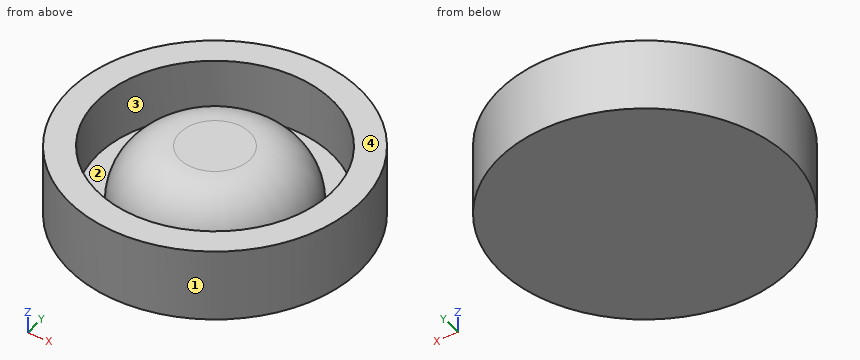
```python
from build123d import *

# Parameters (mm, degrees)
F0_R     = 25.4
F1_DEPTH = 12.7
F2_R     = 20.5279895556
F3_DEPTH = 10.16
F4_R     = 16.2758477469
F5_DEPTH = 10.16
F6_R     = 10.15999


# Not quite as in the source:
# - a fillet or chamfer is up to 0.001 mm smaller than in the source, because OpenCascade refuses the exact size


with BuildPart() as f1:
    # F0 (on Top) → F1 (new body)
    with BuildSketch(Plane.XY):
        Circle(F0_R)
    extrude(amount=F1_DEPTH)

    # F2 (on face) → F3 (cut)
    with BuildSketch(Plane.XY.offset(12.7)):
        Circle(F2_R)
    extrude(amount=-F3_DEPTH, mode=Mode.SUBTRACT)

    # F4 (on face) → F5 (join)
    with BuildSketch(Plane.XY.offset(2.54)):
        Circle(F4_R)
    extrude(amount=F5_DEPTH)

    # F6 (radius 10.16 in the source; OpenCascade refuses exactly that, so slightly less here)
    f6_edges = [f1.edges().sort_by_distance(p)[0] for p in [
        (-16.275848, 0, 12.7),
    ]]
    fillet(f6_edges, radius=F6_R)


solid = f1.part
```
For this review, take the finished solid that the model builds, in its own axes (mm). Face numbers are marked on the shaded views. Round coordinates to 2 decimals unless told otherwise and drop trailing zeros. Loops run counter-clockwise (first coordinate to the right, second up) from the corner with the lowest first, then second, coordinate; pieces in that order, holes last.
Q1. Mouldability with a two-part tool opening along Y and no side actions: class the marked faces 1, 2, 3 and 4 as +Y half, -Y half, draft (parallel to the pull), parting line (faces both ways), or undercut.
Result sheet:
face 1: parting line
face 2: undercut
face 3: undercut
face 4: draft
Q2. Insertion check: pin 1 Ø8 at (x, y) = (-18, -8.5) entering from +Z; pin 2 Ø6 at (y, z) = (-12.5, 8) entering from +X; pin 3 Ø5 at (y, z) = (11.5, 7) entering from -X; pin 4 Ø5 at (y, z) = (-18.5, 2.5) entering from -X. Each pin has a flat end and moves straight along its axis. Give the tip position at first contact, or say it passes through.
Result sheet:
pin 1: stops at z = 12.7
pin 2: stops at x = 23.56
pin 3: stops at x = -23.75
pin 4: stops at x = -19.73
Q3. Add section B-B on z = 8. Give the number of separate pieces and of enclosed holes in the cut face, plus the area to 3 significant figures.
Result sheet:
separate pieces: 2
enclosed holes: 1
area: 1,380 mm2
Q4. Add section A-A on x = -17.5. Write out the cut boundary in (y, z), plus the area to 3 significant figures.
Result sheet:
outline: (-18.41, 0) - (18.41, 0) - (18.41, 12.7) - (10.73, 12.7) - (10.73, 2.54) - (-10.73, 2.54) - (-10.73, 12.7) - (-18.41, 12.7) - close
area: 250 mm2
Q5. To check wall thickness, follow line 1 along Y through (x, z) = (0, 5.75); line 2 along Y through (x, z) = (-4, 6.25); line 3 along X through (y, z) = (-11.5, 10). State the ranges of each line that lie inside material, in increasing order.
Result sheet:
line 1: y = -25.4 to -20.53, -15.76 to 15.76, 20.53 to 25.4
line 2: y = -25.08 to -20.13, -15.05 to 15.05, 20.13 to 25.08
line 3: x = -22.65 to -17, -6.09 to 6.09, 17 to 22.65
